Part model, mm, in its own coordinate system. A direction names the side the tool comes from. Give positions to 0.01 mm unless a question says otherwise; leave off trailing zeros. Loops run counter-clockwise (first coordinate to the right, second up) from the corner with the lowest first, then second, coordinate; pieces in that order, holes last. Notation, with made-up numbers: (45.5, -2) -> (81.5, -2) arc R28 cw to (81.5, 29) -> close; hole circle Ø6 at (68.5, 19). An arc over 180 degrees is marked (long way). Write item = value, one per line.
Autodesk Inventor part; units mm, degrees
ref_plane "YZ Plane" through (0, 0, 0) normal (1, 0, 0) x (0, 1, 0)
ref_plane "XZ Plane" through (0, 0, 0) normal (0, 1, 0) x (-1, 0, 0)
ref_plane "XY Plane" through (0, 0, 0) normal (0, 0, 1) x (1, 0, 0)
sketch "Sketch1" plane through (0, 0, 0) normal (0, 1, 0) x (-1, 0, 0)
  line L0 (0, 0) -> (0, -23.8252)
  line L1 (0, -23.8252) -> (7.7978, -23.8252)
  line L2 (7.7978, -23.8252) -> (7.7978, 0)
  line L3 (7.7978, 0) -> (0, 0)
  dimension "d0" = 23.8252
  dimension "d1" = 7.7978
extrude "Extrusion1" add sketch "Sketch1" along normal blind 3.236
shell "Shell1" thickness 1.4732 removed faces 1 at (-2.5993, 3.236, -7.9417)
sketch "Sketch3" plane through (-6.3246, 1.4732, -22.352) normal (0, 1, 0) x (1, 0, 0)
  point P0 (6.3246, -22.352)
sketch "Sketch4" plane through (-6.3246, 1.4732, -22.352) normal (0, 1, 0) x (1, 0, 0)
  line L0 (6.3246, -22.352) -> (2.4257, -22.352) construction
  line L1 (2.4257, -22.352) -> (2.4257, -18.4531) construction
  line L2 (2.4257, -18.4531) -> (6.3246, -18.4531) construction
  line L3 (6.3246, -18.4531) -> (6.3246, -22.352) construction
  circle A0 centre (2.4257, -18.4531) radius 2.4498 construction
  circle A1 centre (2.4257, -10.6553) radius 2.4498 construction
  line L4 (2.4257, -18.4531) -> (2.4257, -10.6553) construction
  circle A2 centre (2.4257, -14.5542) radius 1.4491
  circle A3 centre (2.4257, -14.5542) radius 0.6198
  dimension "d5" = 3.8989
  dimension "d6" = 3.8989
  dimension "d7" = 4.8997
  dimension "d10" = 7.7978
  dimension "d15" = 1.2395
extrude "Extrusion2" add sketch "Sketch4" along normal up to surface (1.7628 mm away)
pattern_linear "Rectangular Pattern1" count 2 spacing 7.7978 along (0, 0, -1) of "Extrusion2"
properties part number "1x3 short orange smooth" material "ABS Plastic"
1) Pull direction Z, two halves, no side cores. Call faces 1 (the face through (-4, 2, -23.825)), 2 (the face through (-3.23, 2.342, -9.083)), 3 (the face through (-3, 3.236, -16)): pulls with the +Z half, pulls with the -Z half, needs draft (parallel to the pull), parting line crosses it, or undercut.
Resolved:
face_1 = pulls with the -Z half
face_2 = undercut
face_3 = needs draft
2) Drill centre lines: line 1 along Z through (x, y) = (-4.25, 2.1); line 2 along X through (y, z) = (2.9, -10); line 3 along X through (y, z) = (2.55, -8). Where is each one in solid material? Low to high. Write a range as [from, to].
Resolved:
line_1 = [-23.83, -22.35], [-17, -16.11], [-15.08, -14.19], [-9.2, -8.31], [-7.29, -6.39], [-1.47, 0]
line_2 = [-7.8, -6.32], [-1.47, 0]
line_3 = [-7.8, -6.32], [-5.33, -4.48], [-3.31, -2.46], [-1.47, 0]
3) Which spindle directions (+Z, -Z, +X, -X, +Y, -Y) get a long thin tool onto all of the face, cutting with end or side? Do faces 4 (the face through (-4, 2, -22.352)), 5 (the face through (-1, 3.236, -12)). Say none if no direction does.
Resolved:
face_4 = +Y
face_5 = +Z, -Z, +X, -X, +Y
4) Slice it at C-C, the plane z = -13.5. List the corners of the cut face in (x, y), and give its area (3 significant figures).
Resolved:
outline = (-7.8, 0) -> (0, 0) -> (0, 3.24) -> (-1.47, 3.24) -> (-1.47, 1.47) -> (-6.32, 1.47) -> (-6.32, 3.24) -> (-7.8, 3.24) -> close
area = 16.7 mm²
5) Slice it at A-A, the plane y = 2.85. List the corners of the cut face in (x, z).
Resolved:
outline = (-7.8, -23.83) -> (0, -23.83) -> (0, 0) -> (-7.8, 0) -> close; circle Ø2.9 at (-3.9, -15.6); circle Ø2.9 at (-3.9, -7.8); hole (-6.32, -22.35) -> (-1.47, -22.35) -> (-1.47, -1.47) -> (-6.32, -1.47) -> close; hole circle Ø1.24 at (-3.9, -15.6); hole circle Ø1.24 at (-3.9, -7.8)
6) Drop a flat-ended pin along its axis: P1, Ø3, axis at x = -5.5, z = -20.5, coming from the -Y side. Give the stop position or say it passes through.
Resolved:
P1 = 0
7) Slice it at B-B, the plane x = -6. List the corners of the cut face in (y, z), and give its area (3 significant figures).
Resolved:
outline = (0, -23.83) -> (3.24, -23.83) -> (3.24, -22.35) -> (1.47, -22.35) -> (1.47, -1.47) -> (3.24, -1.47) -> (3.24, 0) -> (0, 0) -> close
area = 40.3 mm²
